Verification items for the finished model (mm, model axes). Face numbers are marked on the shaded views. A direction names the side the tool comes from. Coordinates: 2 decimals unless noted, no trailing zeros. Order: outer loops, then holes, each group sorted by start corner. A loop starts at its lowest first (then second) coordinate and runs counter-clockwise, first axis right, second up. Notation, with made-up numbers: M 48,34 L 80,34 A23 cw 80,52 Z; hole C 12,40 d11. An arc over 180 degrees is marked long. Write item = value, one per line.
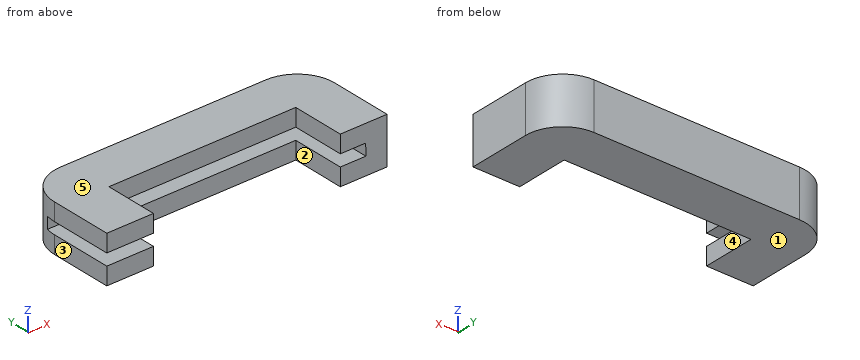
```python
from build123d import *

# Parameters (mm, degrees)
F0_W        = 6.35
F0_H        = 6.35
F0_H_2      = 7.196190767
F1_DEPTH    = 6.35
F2_W        = 6.35
F2_H        = 1.5875
F3_DEPTH    = 9.779
F4_T1_DEPTH = 31.75


# Not quite as in the source:
# - a fillet or chamfer that OpenCascade refuses, or shapes differently, is made with other operations: its cross-section is extruded or revolved along the edge and cut away or added


with BuildPart() as f1:
    # F0 (on Top) → F1 (new body)
    with BuildSketch(Plane.XY):
        Polygon((-12.7, 13.546190767), (-12.7, 7.196190767), (0, 7.196190767), (12.7, 7.196190767), (12.7, 13.546190767), align=None)
        with Locations((-15.875, 10.371190767)):
            Rectangle(F0_W, F0_H)
        with Locations((-15.875, 3.5980953835)):
            Rectangle(F0_W, F0_H_2)
        with Locations((15.875, 10.371190767)):
            Rectangle(F0_W, F0_H)
        with Locations((15.875, 3.5980953835)):
            Rectangle(F0_W, F0_H_2)
    extrude(amount=F1_DEPTH)

    # F2 (on face) → F3 (cut)
    with BuildSketch(Plane.XZ):
        Polygon((9.525, 3.96875), (-8.7374933064, 3.96875), (-12.7, 3.96875), (-12.7, 2.38125), (-8.7374933064, 2.38125), (9.525, 2.38125), align=None)
        Polygon((16.1540079862, 3.96875), (9.525, 3.96875), (9.525, 2.38125), (16.1763634533, 2.38125), align=None)
        with Locations((-15.875, 3.175)):
            Rectangle(F2_W, F2_H)
    extrude(amount=-F3_DEPTH, mode=Mode.SUBTRACT)

    # F4: fillet of radius 5.08 on 2 edges, made by hand

    # F4_s2 → F4_t1 (cut)
    with BuildSketch(Plane.XY.offset(-12.7)):
        with BuildLine():
            ThreePointArc((13.97, 13.546190767), (17.5621024484, 12.0582932154), (19.05, 8.466190767))
            Line((19.05, 8.466190767), (19.05, 13.546190767))
            Line((19.05, 13.546190767), (13.97, 13.546190767))
        make_face()
        with BuildLine():
            ThreePointArc((-19.05, 8.466190767), (-17.5621024484, 12.0582932154), (-13.97, 13.546190767))
            Line((-13.97, 13.546190767), (-19.05, 13.546190767))
            Line((-19.05, 13.546190767), (-19.05, 8.466190767))
        make_face()
    extrude(amount=F4_T1_DEPTH, mode=Mode.SUBTRACT)


solid = f1.part
```
Item 1: Sectioned sample at B-B, the plane z = 2. Enter the section's corners in (x, y), then the cut area to 3 significant figures.
Report:
outline = M -19.05,0 L -12.7,0 L -12.7,7.2 L 12.7,7.2 L 12.7,0 L 19.05,0 L 19.05,8.47 A5.08 ccw 13.97,13.55 L -13.97,13.55 A5.08 ccw -19.05,8.47 Z
area = 322 mm^2
Item 2: Scan lines: L1, parallel to X at y = 4, z = 1.5; L2, parallel to Z at x = -12, y = 8.75; L3, parallel to X at y = 2.5, z = 2.5. Record each from-to range of solid material in increasing order. Write a range as from..to.
Report:
L1 = -19.05..-12.7, 12.7..19.05
L2 = 0..2.38, 3.97..6.35
L3 = 16.17..19.05
Item 3: Sectioned sample at C-C, the plane x = -9. Enter the section's corners in (y, z), then the cut area to 3 significant figures.
Report:
outline = M 7.2,0 L 13.55,0 L 13.55,6.35 L 7.2,6.35 L 7.2,3.97 L 9.78,3.97 L 9.78,2.38 L 7.2,2.38 Z
area = 36.2 mm^2
Item 4: Sectioned sample at A-A, the plane y = 1.5. Enter the section's corners in (x, z).
Report:
outline = M -19.05,0 L -12.7,0 L -12.7,2.38 L -19.05,2.38 Z; M -19.05,3.97 L -12.7,3.97 L -12.7,6.35 L -19.05,6.35 Z; M 12.7,0 L 19.05,0 L 19.05,6.35 L 12.7,6.35 L 12.7,3.97 L 16.15,3.97 L 16.18,2.38 L 12.7,2.38 Z
Item 5: Release check for a two-part mould opening along X. For the marked faces 3, 4 and 5 record: pulls with the +X half, pulls with the -X half, needs draft (parallel to the pull), parting line crosses it, or undercut.
Report:
face_3 = pulls with the -X half
face_4 = undercut
face_5 = needs draft
Item 6: Gauge pin test, flat ends, axial feed: pin 1 (0.8 mm diameter, centred on x = -6.5, z = 3.5, fed in from -Y); pin 2 (0.7 mm diameter, centred on x = -1.5, z = 1.5, fed in from -Y). Record the tip position at first contact, or that the pin passes through.
Report:
pin_1 = 9.78
pin_2 = 7.2
Item 7: Sectioned sample at D-D, the plane y = 8. Enter the section's corners in (x, z).
Report:
outline = M -19.05,0 L 19.05,0 L 19.05,6.35 L -19.05,6.35 L -19.05,3.97 L 16.15,3.97 L 16.18,2.38 L -19.05,2.38 Z
Item 8: Tool access check on the marked faces 1 and 2. Record the directions out of +Z, -Z, +X, -X, +Y, -Y that give a thin tool (end or side, any length) a straight path to the whole face; none if there is none.
Report:
face_1 = -Z, +X, -X, +Y, -Y
face_2 = +Z, -Z, -Y
